```python
from build123d import *

# Parameters (mm, degrees)
SKETCH1_R           = 3.175
BOSS_EXTRUDE1_DEPTH = 75
SKETCH2_R           = 34.925
BOSS_EXTRUDE2_DEPTH = 5


with BuildPart() as part:
    # Sketch1 → Boss-Extrude1 (new body, symmetric)
    with BuildSketch(Plane(origin=(0, 0, 0), x_dir=(0, 0, -1), z_dir=(1, 0, 0))):
        Circle(SKETCH1_R)
    extrude(amount=BOSS_EXTRUDE1_DEPTH, both=True)

    # Sketch2 → Boss-Extrude2 (add)
    with BuildSketch(Plane(origin=(75, 0, 0), x_dir=(0, 0, -1), z_dir=(1, 0, 0))):
        Circle(SKETCH2_R)
    boss_extrude2 = extrude(amount=BOSS_EXTRUDE2_DEPTH)

    # Mirror1: Boss-Extrude2 across plane
    add(boss_extrude2.mirror(Plane(origin=(0, 0, 0), x_dir=(0, 0, 1), z_dir=(1, 0, 0))))


solid = part.part
```
Can you work these out from the model? Positions are in its coordinate system, mm. Round coordinates to 2 decimals unless told otherwise and drop trailing zeros. Loops run counter-clockwise (first coordinate to the right, second up) from the corner with the lowest first, then second, coordinate; pieces in that order, holes last. Notation, with made-up numbers: M 20.5,68 L 36.5,68 A11 ccw 36.5,88 Z; hole C 66,-2 d4. An arc over 180 degrees is marked long. Write item = value, one per line. Start each with the question number.
(1) Suppose I cut it at A-A on y = -12.5. Write out the boundary of the cut face in (x, z).
(2) Suppose I cut it at B-B on z = -28. Write out the boundary of the cut face in (x, y).
(3) I'm going to push flat-ended pins straight in: P1, Ø2, axis at x = 40.5, z = -1.5, coming from the -Y side; P2, Ø12, axis at x = 24.5, z = -11, coming from the +Y side; P3, Ø5, axis at x = 2.5, z = -0.5, coming from the +Y side (3 decimals). Where does each tip first touch, or does it pass through?
(4) If we mould it in two halves opening along X, with no side actions, what happens to faces 1 (the face through (1.05, -3.1, 0.69)), 2 (the face through (75, 0, -7)), 3 (the face through (80, 0, 0)), 4 (the face through (77.465, -21.251, 27.715))? For each: released by +X, released by -X, zero draft, split by the parting line, or undercut.
(5) Suppose I cut it at C-C on z = 0. Write out the boundary of the cut face in (x, y) (3 decimals).
(6) I need wall thicknesses on line 1 along X through (y, z) = (-31, 4); line 2 along Z through (x, y) = (32, 1.5); line 3 along Z through (x, y) = (-4, 1). Which ranges of each line are inside material? Lowest first, please.
Answer block:
q1.outline = M -80,-32.61 L -75,-32.61 L -75,32.61 L -80,32.61 Z; M 75,-32.61 L 80,-32.61 L 80,32.61 L 75,32.61 Z
q2.outline = M -80,-20.87 L -75,-20.87 L -75,20.87 L -80,20.87 Z; M 75,-20.87 L 80,-20.87 L 80,20.87 L 75,20.87 Z
q3.P1 = -3.14
q3.P2 = through
q3.P3 = 3.175
q4.face_1 = undercut
q4.face_2 = undercut
q4.face_3 = released by +X
q4.face_4 = zero draft
q5.outline = M -80,-34.925 L -75,-34.925 L -75,-3.175 L 75,-3.175 L 75,-34.925 L 80,-34.925 L 80,34.925 L 75,34.925 L 75,3.175 L -75,3.175 L -75,34.925 L -80,34.925 Z
q6.line_1 = -80 to -75, 75 to 80
q6.line_2 = -2.8 to 2.8
q6.line_3 = -3.01 to 3.01
